The listing builds one solid part. Answer for the finished solid, in the listing's coordinates (mm). Give positions to 0.01 mm unless a question says otherwise; leave off trailing zeros. Order: outer loops, then holes, each group sorted by start corner. A loop starts at its lowest first (then second) coordinate and runs counter-clockwise, first axis right, second up. Notation, with made-up numbers: (16.5, 51) - (46.5, 51) arc R31 cw to (46.5, 85) - close; hole circle Ø4 at (-12, 88). An arc over 180 degrees is marked (long way). Answer as CSV lines item,"result". Start each with the question number.
1. Flat-ended cylindrical pins translate along their axes: pin 1 (8 mm diameter, centred on x = 76, y = 20, fed in from -Z); pin 2 (1.5 mm diameter, centred on y = 17.5, z = 2, fed in from +X); pin 3 (6 mm diameter, centred on x = 83, z = -1, fed in from -Y). Find the tip coordinate at first contact, or state that the pin passes through.
2. Consider line 1 along Y through (x, z) = (0, 2.65); line 2 along Y through (x, z) = (57, 1.5); line 3 along Z through (x, y) = (12, -4). Determine where each line is inside the solid, lowest interval first. Write a range as [from, to].
3. Section C-C on x = -75 is taken. Give the vertices of the cut face in (y, z).
4. Section B-B on y = 68 is taken. Give the vertices of the cut face in (x, z).
5. Section A-A on x = 0 is taken. Give the vertices of the cut face in (y, z), and give its area (3 significant figures).
6. Section D-D on z = -5.75 is taken. Give the vertices of the cut face in (x, y), and give its area (3 significant figures).
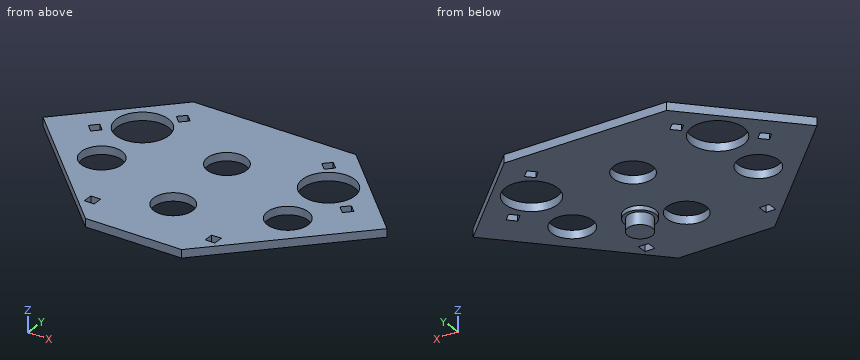
from build123d import *

# Parameters (mm, degrees)
SKETCH3_R           = 12
BOSS_EXTRUDE1_DEPTH = 5
BOSS_EXTRUDE2_DEPTH = 5
SKETCH6_R           = 16
SKETCH6_R_2         = 12.5
SKETCH6_W           = 6
SKETCH6_H           = 6
CUT_EXTRUDE1_DEPTH  = 5
SKETCH7_R           = 7.5
BOSS_EXTRUDE3_DEPTH = 10
SKETCH8_R           = 9.5
SKETCH8_R_2         = 7.5
BOSS_EXTRUDE4_DEPTH = 2.5


with BuildPart() as part:
    # Sketch3 → Boss-Extrude1 (new body)
    with BuildSketch(Plane.XY):
        Polygon((-77.781745931, 49.497474683), (-49.497474683, 77.781745931), (-43.840620434, 83.43860018), (43.840620434, 83.43860018), (49.497474683, 77.781745931), (77.781745931, 49.497474683), (88.388347648, 38.890872965), (27.497474683, -22), (-27.497474683, -22), (-88.388347648, 38.890872965), align=None)
        Circle(SKETCH3_R, mode=Mode.SUBTRACT)
        with Locations((0, 50)):
            Circle(SKETCH3_R, mode=Mode.SUBTRACT)
        Polygon((-81.317279836, 44.547727215), (-77.074639149, 48.790367902), (-72.831998462, 44.547727215), (-77.074639149, 40.305086528), align=None, mode=Mode.SUBTRACT)
        Polygon((-48.790367902, 77.074639149), (-44.547727215, 81.317279836), (-40.305086528, 77.074639149), (-44.547727215, 72.831998462), align=None, mode=Mode.SUBTRACT)
        Polygon((40.305086528, 77.074639149), (44.547727215, 72.831998462), (48.790367902, 77.074639149), (44.547727215, 81.317279836), align=None, mode=Mode.SUBTRACT)
        Polygon((72.831998462, 44.547727215), (77.074639149, 40.305086528), (81.317279836, 44.547727215), (77.074639149, 48.790367902), align=None, mode=Mode.SUBTRACT)
    extrude(amount=BOSS_EXTRUDE1_DEPTH)

    # Sketch5 → Boss-Extrude2 (add)
    with BuildSketch(Plane.XY.offset(5)):
        Polygon((-105.358910397, 38.890872965), (-49.811183182, 94.43860018), (49.811183182, 94.43860018), (105.358910397, 38.890872965), (29.468037432, -37), (-29.468037432, -37), align=None)
        Polygon((-43.840620434, 83.43860018), (-88.388347648, 38.890872965), (-27.497474683, -22), (27.497474683, -22), (88.388347648, 38.890872965), (43.840620434, 83.43860018), align=None, mode=Mode.SUBTRACT)
    extrude(amount=-BOSS_EXTRUDE2_DEPTH)

    # Sketch6 → Cut-Extrude1 (cut)
    with BuildSketch(Plane.XY.offset(5)):
        with Locations((-57, 58)):
            Circle(SKETCH6_R)
        with Locations((-57, 20)):
            Circle(SKETCH6_R_2)
        with Locations(Location((57, 20, 0), (0, 0, 180))):
            Circle(SKETCH6_R_2)
        with Locations(Location((57, 58, 0), (0, 0, 180))):
            Circle(SKETCH6_R)
        with Locations((-37, -19)):
            Rectangle(SKETCH6_W, SKETCH6_H)
        with Locations((37, -19)):
            Rectangle(SKETCH6_W, SKETCH6_H)
    extrude(amount=-CUT_EXTRUDE1_DEPTH, mode=Mode.SUBTRACT)

    # Sketch7 → Boss-Extrude3 (add)
    with BuildSketch(Plane.XY):
        with Locations((21.11953, 11.4)):
            Circle(SKETCH7_R)
    extrude(amount=-BOSS_EXTRUDE3_DEPTH)

    # Sketch8 → Boss-Extrude4 (add)
    with BuildSketch(Plane(origin=(0, 0, 0), x_dir=(-1, 0, 0), z_dir=(0, 0, -1))):
        with Locations((-21.11953, 11.4)):
            Circle(SKETCH8_R)
        with Locations(Location((-21.11953, 11.4, 0), (0, 0, 180))):
            Circle(SKETCH8_R_2, mode=Mode.SUBTRACT)
    extrude(amount=BOSS_EXTRUDE4_DEPTH)


solid = part.part
Checks:
1,pin 1,"stops at z = 0"
1,pin 2,"stops at x = 84.72"
1,pin 3,"stops at y = 13.7"
2,line 1,"y = [-37, -12], [12, 38], [62, 94.44]"
2,line 2,"y = [-9.47, 7.5], [32.5, 42], [74, 87.25]"
2,line 3,"z = [0, 5]"
3,outline,"(8.53, 0) - (42.38, 0) - (42.38, 5) - (8.53, 5) - close; (46.72, 0) - (69.25, 0) - (69.25, 5) - (46.72, 5) - close"
4,outline,"(-76.25, 0) - (-69.49, 0) - (-69.49, 5) - (-76.25, 5) - close; (-44.51, 0) - (44.51, 0) - (44.51, 5) - (-44.51, 5) - close; (69.49, 0) - (76.25, 0) - (76.25, 5) - (69.49, 5) - close"
5,outline,"(-37, 0) - (-12, 0) - (-12, 5) - (-37, 5) - close; (12, 0) - (38, 0) - (38, 5) - (12, 5) - close; (62, 0) - (94.44, 0) - (94.44, 5) - (62, 5) - close"
5,area,"417 mm²"
6,outline,"circle Ø15 at (21.12, 11.4)"
6,area,"177 mm²"
